```python
from build123d import *

# Parameters (mm, degrees)
BOSS_EXTRUDE1_DEPTH = 105
SKETCH3_W           = 54
SKETCH3_H           = 102
BOSS_EXTRUDE2_DEPTH = 2
BOSS_EXTRUDE3_START = -105
SKETCH3_2_W         = 54
SKETCH3_2_H         = 102
BOSS_EXTRUDE3_DEPTH = 2
BOSS_EXTRUDE4_DEPTH = 3.5
CHAMFER1_SIZE       = 0.5
SKETCH5_W           = 15
SKETCH5_H           = 50
CUT_EXTRUDE1_DEPTH  = 158.381701605
SKETCH7_W           = 6
SKETCH7_H           = 25
CUT_EXTRUDE2_DEPTH  = 158.381701605
FILLET1_R           = 2
CHAMFER2_SIZE       = 1.5
SKETCH8_R           = 1.5
SKETCH8_W           = 7.2
SKETCH8_H           = 7.7
SKETCH8_H_2         = 10.7
CUT_EXTRUDE3_DEPTH  = 158.381701605


with BuildPart() as part:
    # Sketch1 → Boss-Extrude1 (new body)
    with BuildSketch(Plane(origin=(0, 0, 0), x_dir=(0, 0, -1), z_dir=(1, 0, 0))):
        Polygon((0, 0), (54, 0), (54, 102), (52, 102), (52, 2), (0, 2), align=None)
    extrude(amount=BOSS_EXTRUDE1_DEPTH)

    # Sketch3 → Boss-Extrude2 (add)
    with BuildSketch(Plane(origin=(105, 0, 0), x_dir=(0, 0, -1), z_dir=(1, 0, 0))):
        with Locations((27, 51)):
            Rectangle(SKETCH3_W, SKETCH3_H)
    extrude(amount=BOSS_EXTRUDE2_DEPTH)

    # Sketch3<2> → Boss-Extrude3 (add)
    with BuildSketch(Plane(origin=(105, 0, 0), x_dir=(0, 0, -1), z_dir=(1, 0, 0)).offset(BOSS_EXTRUDE3_START)):
        with Locations((27, 51)):
            Rectangle(SKETCH3_2_W, SKETCH3_2_H)
    extrude(amount=-BOSS_EXTRUDE3_DEPTH)

    # Sketch4 → Boss-Extrude4 (add)
    with BuildSketch(Plane.XZ.offset(-2)):
        Polygon((42.6, -4.5), (39.6, -7.5), (35.6, -7.5), (32.6, -4.5), align=None)
        Polygon((17.6, -4.5), (14.6, -7.5), (10.6, -7.5), (7.6, -4.5), align=None)
        Polygon((67.6, -4.5), (64.6, -7.5), (60.6, -7.5), (57.6, -4.5), align=None)
    extrude(amount=-BOSS_EXTRUDE4_DEPTH)

    # Chamfer1
    chamfer1_edges = [part.edges().sort_by_distance(p)[0] for p in [
        (12.6, 5.5, -4.5),
        (16.1, 5.5, -6),
        (12.6, 5.5, -7.5),
        (9.1, 5.5, -6),
        (37.6, 5.5, -4.5),
        (41.1, 5.5, -6),
        (37.6, 5.5, -7.5),
        (34.1, 5.5, -6),
        (62.6, 5.5, -4.5),
        (66.1, 5.5, -6),
        (62.6, 5.5, -7.5),
        (59.1, 5.5, -6),
    ]]
    chamfer(chamfer1_edges, length=CHAMFER1_SIZE)

    # Sketch5 → Cut-Extrude1 (cut, through all)
    with BuildSketch(Plane(origin=(0, 0, -54), x_dir=(-1, 0, 0), z_dir=(0, 0, -1))):
        with Locations((-42.7, 37)):
            Rectangle(SKETCH5_W, SKETCH5_H)
        with Locations((-17.7, 37)):
            Rectangle(SKETCH5_W, SKETCH5_H)
        with Locations((-67.7, 37)):
            Rectangle(SKETCH5_W, SKETCH5_H)
    extrude(amount=-CUT_EXTRUDE1_DEPTH, mode=Mode.SUBTRACT)

    # Sketch7 → Cut-Extrude2 (cut, through all)
    with BuildSketch(Plane.XZ):
        with Locations((20.7, -31.5)):
            Rectangle(SKETCH7_W, SKETCH7_H)
        with Locations((45.7, -31.5)):
            Rectangle(SKETCH7_W, SKETCH7_H)
        with Locations((70.7, -31.5)):
            Rectangle(SKETCH7_W, SKETCH7_H)
    extrude(amount=-CUT_EXTRUDE2_DEPTH, mode=Mode.SUBTRACT)

    # Fillet1
    fillet1_edges = [part.edges().sort_by_distance(p)[0] for p in [
        (25.2, 12, -53),
        (25.2, 62, -53),
        (10.2, 62, -53),
        (10.2, 12, -53),
        (50.2, 62, -53),
        (35.2, 62, -53),
        (35.2, 12, -53),
        (50.2, 12, -53),
        (75.2, 62, -53),
        (60.2, 62, -53),
        (60.2, 12, -53),
        (75.2, 12, -53),
    ]]
    fillet(fillet1_edges, radius=FILLET1_R)

    # Chamfer2
    chamfer2_edges = [part.edges().sort_by_distance(p)[0] for p in [
        (17.7, 1, -44),
        (17.7, 1, -19),
        (23.7, 1, -19),
        (23.7, 1, -44),
        (48.7, 1, -44),
        (42.7, 1, -44),
        (42.7, 1, -19),
        (48.7, 1, -19),
        (73.7, 1, -44),
        (67.7, 1, -44),
        (67.7, 1, -19),
        (73.7, 1, -19),
    ]]
    chamfer(chamfer2_edges, length=CHAMFER2_SIZE)

    # Sketch8 → Cut-Extrude3 (cut, through all)
    with BuildSketch(Plane(origin=(0, 0, 0), x_dir=(-1, 0, 0), z_dir=(0, -1, 0))):
        with Locations(Location((-83.7, 18, 0), (0, 0, 90))):
            Circle(SKETCH8_R)
        with Locations(Location((-83.7, 38.5, 0), (0, 0, 90))):
            Circle(SKETCH8_R)
        with BuildLine():
            Line((-81.9, 36.35), (-85.5, 36.35))
            ThreePointArc((-85.5, 36.35), (-87.267766953, 35.617766953), (-88, 33.85))
            Line((-88, 33.85), (-88, 20.15))
            Line((-88, 20.15), (-79.4, 20.15))
            Line((-79.4, 20.15), (-79.4, 33.85))
            ThreePointArc((-79.4, 33.85), (-80.132233047, 35.617766953), (-81.9, 36.35))
        make_face()
        with Locations((-98, 18)):
            Rectangle(SKETCH8_W, SKETCH8_H)
        with Locations((-98, 36)):
            Rectangle(SKETCH8_W, SKETCH8_H_2)
    extrude(amount=-CUT_EXTRUDE3_DEPTH, mode=Mode.SUBTRACT)


solid = part.part
```
Verification items for the finished model (mm, model axes). A direction names the side the tool comes from. Round coordinates to 2 decimals unless told otherwise and drop trailing zeros. Write each loop counter-clockwise with the first axis right and the second up, starting at its lowest first coordinate (ties: lowest second). Pieces come first, ordered by that corner, then holes. Notation, with made-up numbers: (7.5, 24) -> (27.5, 24) arc R22 cw to (27.5, 49) -> close; hole circle Ø6 at (89.25, 11). An arc over 180 degrees is marked (long way). Write each question's results on one line, items separated by ' | '.
Q1. Draft check along X on faces 4 (the face through (53, 0, -27)), 5 (the face through (87.248, 0.986, -35.637)). Enter one of: released by +X, released by -X, zero draft, split by the parting line, or undercut.
Derived:
face 4: zero draft | face 5: undercut
Q2. Access from +Z, -Z, +X, -X, +Y, -Y to the whole of each face (thin tool, end or side, straight path). Record for faces 1 (the face through (59.63, 5.25, -6.18)), 2 (the face through (77, 1.7, 0)), 3 (the face through (105, 53, -26)).
Derived:
face 1: +Y | face 2: +Z, +X, -X, +Y, -Y | face 3: +Z, +Y
Q3. Thickness scan on probe 1 along X at (y, z) = (1.65, -38.5); probe 2 along X at (y, z) = (0.5, -18); probe 3 along X at (y, z) = (41.5, -12). Record the ranges inside material, lowest first.
Derived:
probe 1: x = -2 to 17.7, 23.7 to 42.7, 48.7 to 67.7, 73.7 to 82.2, 85.2 to 94.4, 101.6 to 107 | probe 2: x = -2 to 82.2, 85.2 to 94.4, 101.6 to 107 | probe 3: x = -2 to 0, 105 to 107
Q4. Sectioned sample at C-C, the plane x = 83.7. Record the boundary of the cut face in (y, z).
Derived:
outline: (0, -54) -> (102, -54) -> (102, -52) -> (2, -52) -> (2, -40) -> (0, -40) -> close; (0, -37) -> (2, -37) -> (2, -36.35) -> (0, -36.35) -> close; (0, -20.15) -> (2, -20.15) -> (2, -19.5) -> (0, -19.5) -> close; (0, -16.5) -> (2, -16.5) -> (2, 0) -> (0, 0) -> close
Q5. Sectioned sample at D-D, the plane y = 37.5. Record the boundary of the cut face in (x, z).
Derived:
outline: (-2, -54) -> (10.2, -54) -> (10.2, -52) -> (0, -52) -> (0, 0) -> (-2, 0) -> close; (25.2, -54) -> (35.2, -54) -> (35.2, -52) -> (25.2, -52) -> close; (50.2, -54) -> (60.2, -54) -> (60.2, -52) -> (50.2, -52) -> close; (75.2, -54) -> (107, -54) -> (107, 0) -> (105, 0) -> (105, -52) -> (75.2, -52) -> close
Q6. Go/stop test with flat-tipped pins: pin 1 Ø2.5 at (x, y) = (10.5, 3.5) entering from +Z; pin 2 Ø5 at (x, z) = (83.7, -38.5) entering from -Y; pin 3 Ø0.6 at (x, z) = (62.5, -5.5) entering from +Y; pin 4 Ø8 at (x, z) = (65, -26.5) entering from +Y. Record where each tip stops, or that it passes through.
Derived:
pin 1: stops at z = -4.5 | pin 2: stops at y = 0 | pin 3: stops at y = 5.5 | pin 4: stops at y = 2
Q7. Sectioned sample at B-B, the plane z = -25.5. Record the boundary of the cut face in (x, y).
Derived:
outline: (-2, 0) -> (17.7, 0) -> (17.7, 2) -> (0, 2) -> (0, 102) -> (-2, 102) -> close; (23.7, 0) -> (42.7, 0) -> (42.7, 2) -> (23.7, 2) -> close; (48.7, 0) -> (67.7, 0) -> (67.7, 2) -> (48.7, 2) -> close; (73.7, 0) -> (79.4, 0) -> (79.4, 2) -> (73.7, 2) -> close; (88, 0) -> (107, 0) -> (107, 102) -> (105, 102) -> (105, 2) -> (88, 2) -> close
Q8. Sectioned sample at A-A, the plane z = -38.5. Record the boundary of the cut face in (x, y), and give its area (3 significant figures).
Derived:
outline: (-2, 0) -> (17.7, 0) -> (17.7, 2) -> (0, 2) -> (0, 102) -> (-2, 102) -> close; (23.7, 0) -> (42.7, 0) -> (42.7, 2) -> (23.7, 2) -> close; (48.7, 0) -> (67.7, 0) -> (67.7, 2) -> (48.7, 2) -> close; (73.7, 0) -> (82.2, 0) -> (82.2, 2) -> (73.7, 2) -> close; (85.2, 0) -> (94.4, 0) -> (94.4, 2) -> (85.2, 2) -> close; (101.6, 0) -> (107, 0) -> (107, 102) -> (105, 102) -> (105, 2) -> (101.6, 2) -> close | area: 562 mm²
